Geometry check sheet. Reference: the model listing, model coordinates, mm. Face numbers are marked on the shaded views. A direction names the side the tool comes from. Round coordinates to 2 decimals unless told otherwise and drop trailing zeros. Loops run counter-clockwise (first coordinate to the right, second up) from the corner with the lowest first, then second, coordinate; pieces in that order, holes last.
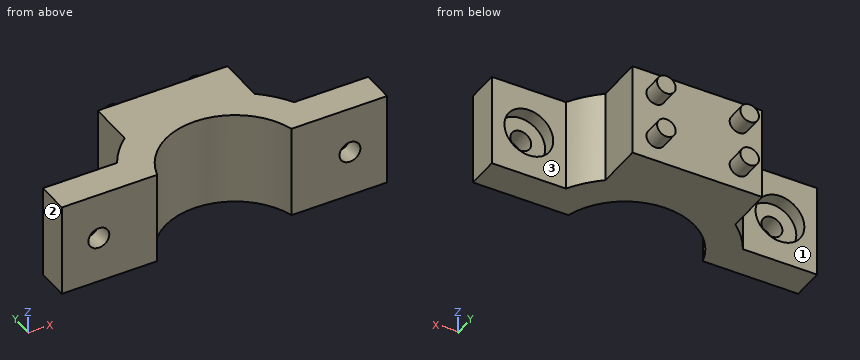
```python
from build123d import *

# Parameters (mm, degrees)
F1_DEPTH = 10
F2_R     = 2.25
F3_DEPTH = 25
F4_R     = 5.25
F4_R_2   = 2.25
F5_DEPTH = 3
F6_W     = 27.92848
F6_H     = 10
F7_DEPTH = 20
F8_R     = 2
F9_DEPTH = 4


with BuildPart() as f1:
    # F0 (on Top) → F1 (new body, symmetric)
    with BuildSketch(Plane.XY):
        with BuildLine():
            Line((-35, 7), (-35, 0))
            Line((-35, 0), (-14.456832, 0))
            ThreePointArc((-14.456832, 0), (0, 11), (14.456832, 0))
            Line((14.456832, 0), (35, 0))
            Line((35, 0), (35, 7))
            Line((35, 7), (19.052559, 7))
            ThreePointArc((19.052559, 7), (0, 18), (-19.052559, 7))
            Line((-19.052559, 7), (-35, 7))
        make_face()
    extrude(amount=F1_DEPTH, both=True)

    # F2 (on face) → F3 (cut)
    with BuildSketch(Plane(origin=(0, 7, 0), x_dir=(-1, 0, 0), z_dir=(0, 1, 0))):
        with Locations((-27.026279, 0)):
            Circle(F2_R)
        with Locations((27.026279, 0)):
            Circle(F2_R)
    extrude(amount=-F3_DEPTH, mode=Mode.SUBTRACT)

    # F4 (on face) → F5 (cut)
    with BuildSketch(Plane(origin=(0, 7, 0), x_dir=(-1, 0, 0), z_dir=(0, 1, 0))):
        with Locations((27.026279, 0)):
            Circle(F4_R)
        with Locations((27.026279, 0)):
            Circle(F4_R_2, mode=Mode.SUBTRACT)
        with Locations((-27.026279, 0)):
            Circle(F4_R)
    extrude(amount=-F5_DEPTH, mode=Mode.SUBTRACT)

    # F6 (on face) → F7 (join)
    with BuildSketch(Plane.XY.offset(10)):
        with Locations((0, 18)):
            Rectangle(F6_W, F6_H)
    extrude(amount=-F7_DEPTH)

    # F8 (on face) → F9 (join)
    with BuildSketch(Plane(origin=(0, 23, 0), x_dir=(-1, 0, 0), z_dir=(0, 1, 0))):
        with Locations((8.96424, -5)):
            Circle(F8_R)
        with Locations((-8.96424, -5)):
            Circle(F8_R)
        with Locations((8.96424, 5)):
            Circle(F8_R)
        with Locations((-8.96424, 5)):
            Circle(F8_R)
    extrude(amount=F9_DEPTH)


solid = f1.part
```
1) Access from +Z, -Z, +X, -X, +Y, -Y to the whole of each face (thin tool, end or side, straight path). Record for the marked faces 1, 2 and 3.
Report:
face 1: +Z, -Z, -X, +Y
face 2: +Z, -Z, -X, +Y, -Y
face 3: +Z, -Z, +X, +Y
2) Gauge pin test, flat ends, axial feed: pin 1 (5 mm diameter, centred on x = 27.03, z = 0, fed in from +Y); pin 2 (5 mm diameter, centred on y = 16, z = -1.5, fed in from +X); pin 3 (3 mm diameter, centred on y = 17.5, z = -2, fed in from -X); pin 4 (4 mm diameter, centred on x = -27.03, z = 0, fed in from -Y). Record the tip position at first contact, or that the pin passes through.
Report:
pin 1: stops at y = 4
pin 2: stops at x = 13.96
pin 3: stops at x = -13.96
pin 4: passes through
3) Sectioned sample at D-D, the plane x = 0. Record the cut outline in (y, z).
Report:
outline: (11, -10) - (23, -10) - (23, 10) - (11, 10) - close
4) Scan lines: line 1 along Y through (x, z) = (24, 6); line 2 along X through (y, z) = (20, -1.25); line 3 along Y through (x, z) = (-29, 2.5). Record each from-to range of solid material in increasing order.
Report:
line 1: y = 0 to 7
line 2: x = -13.96 to 13.96
line 3: y = 0 to 4
5) Sectioned sample at C-C, the plane y = 9. Record the cut outline in (x, z).
Report:
outline: (-17.75, -10) - (-7.48, -10) - (-7.48, 10) - (-17.75, 10) - close; (7.48, -10) - (17.75, -10) - (17.75, 10) - (7.48, 10) - close
6) Sectioned sample at B-B, the plane z = 8.5. Record the cut outline in (x, y), then the cut area to 3 significant figures.
Report:
outline: (-35, 0) - (-14.46, 0) arc R15 cw to (14.46, 0) - (35, 0) - (35, 7) - (19.05, 7) arc R22 ccw to (13.96, 13) - (13.96, 23) - (-13.96, 23) - (-13.96, 13) arc R22 ccw to (-19.05, 7) - (-35, 7) - close
area: 736 mm2
7) Sectioned sample at A-A, the plane z = 0. Record the cut outline in (x, y), then the cut area to 3 significant figures.
Report:
outline: (-35, 0) - (-29.28, 0) - (-29.28, 4) - (-32.28, 4) - (-32.28, 7) - (-35, 7) - close; (-24.78, 0) - (-14.46, 0) arc R15 cw to (14.46, 0) - (24.78, 0) - (24.78, 4) - (21.78, 4) - (21.78, 7) - (19.05, 7) arc R22 ccw to (13.96, 13) - (13.96, 23) - (-13.96, 23) - (-13.96, 13) arc R22 ccw to (-19.05, 7) - (-21.78, 7) - (-21.78, 4) - (-24.78, 4) - close; (29.28, 0) - (35, 0) - (35, 7) - (32.28, 7) - (32.28, 4) - (29.28, 4) - close
area: 637 mm2
